The listing builds one solid part. Answer for the finished solid, in the listing's coordinates (mm). A direction names the side the tool comes from. Round coordinates to 2 decimals unless told otherwise and drop trailing zeros. Write each loop counter-clockwise with the first axis right and the second up, starting at its lowest first coordinate (ties: lowest second). Pieces come first, ordered by that corner, then holes.
from build123d import *

# Parameters (mm, degrees)
EXTRUDE_START             = -26
SKETCH_1_W                = 14
SKETCH_1_H                = 1.5
EXTRUDE_241_DEPTH         = 52
SKETCH_2_W                = 5
SKETCH_2_H                = 3
EXTRUDE_321_DEPTH         = 8
SKETCH_3_R                = 3
EXTRUDE_392_DEPTH         = 8
EXTRUDE_START_2           = 18
SKETCH_4_W                = 5
SKETCH_4_H                = 3
EXTRUDE_4_DEPTH           = 8
SKETCH_5_R                = 3
EXTRUDE_5_DEPTH           = 8
D3P2_START                = -28
SKETCH_6_R                = 1.6
D3P2_DEPTH                = 56
CUT_EXTRUDE_M3_DEPTH      = 100
CUT_EXTRUDE_M3_DEPTH_BACK = 100
SKETCH_7_R                = 1.6
CUT_EXTRUDE_3_DEPTH       = 100
CUT_EXTRUDE_3_DEPTH_BACK  = 100
SKETCH_8_R                = 1.6


with BuildPart() as part:
    # 草图1 → Extrude 241 (new body)
    with BuildSketch(Plane.XY.offset(EXTRUDE_START)):
        with Locations((-11, -2.25)):
            Rectangle(SKETCH_1_W, SKETCH_1_H)
    extrude(amount=EXTRUDE_241_DEPTH)

    # 草图2 → Extrude 321 (add)
    with BuildSketch(Plane.XY.offset(EXTRUDE_START)):
        with Locations((-2.5, -1.5)):
            Rectangle(SKETCH_2_W, SKETCH_2_H)
    extrude(amount=EXTRUDE_321_DEPTH)

    # 草图3 → Extrude 392 (add)
    with BuildSketch(Plane.XY.offset(EXTRUDE_START)):
        Circle(SKETCH_3_R)
    extrude(amount=EXTRUDE_392_DEPTH)

    # 草图4 → 凸台-拉伸4 (add)
    with BuildSketch(Plane.XY.offset(EXTRUDE_START_2)):
        with Locations((-2.5, -1.5)):
            Rectangle(SKETCH_4_W, SKETCH_4_H)
    extrude(amount=EXTRUDE_4_DEPTH)

    # 草图5 → 凸台-拉伸5 (add)
    with BuildSketch(Plane.XY.offset(EXTRUDE_START_2)):
        Circle(SKETCH_5_R)
    extrude(amount=EXTRUDE_5_DEPTH)

    # 草图6 → D3p2转轴通孔 (cut)
    with BuildSketch(Plane.XY.offset(D3P2_START)):
        Circle(SKETCH_6_R)
    extrude(amount=D3P2_DEPTH, mode=Mode.SUBTRACT)

    # 草图7 → 底板M3安装孔 (cut, two sides: drawn at the far end of the back side and taken through both)
    with BuildSketch(Plane(origin=(0, 0, 0), x_dir=(1, 0, 0), z_dir=(0, 1, 0)).offset(-CUT_EXTRUDE_M3_DEPTH_BACK)):
        with Locations(Location((-12, 22, 0), (0, 0, 270))):
            Circle(SKETCH_7_R)
    extrude(amount=CUT_EXTRUDE_M3_DEPTH + CUT_EXTRUDE_M3_DEPTH_BACK, mode=Mode.SUBTRACT)

    # 草图8 → 切除-拉伸3 (cut, two sides: drawn at the far end of the back side and taken through both)
    with BuildSketch(Plane(origin=(0, 0, 0), x_dir=(1, 0, 0), z_dir=(0, 1, 0)).offset(-CUT_EXTRUDE_3_DEPTH_BACK)):
        with Locations(Location((-12, -22, 0), (0, 0, 270))):
            Circle(SKETCH_8_R)
    extrude(amount=CUT_EXTRUDE_3_DEPTH + CUT_EXTRUDE_3_DEPTH_BACK, mode=Mode.SUBTRACT)


solid = part.part
1. For a pull along X with two mould halves and no side action, classify faces 1 (the face through (-13.42, -2.26, 22.74)), 2 (the face through (-1.27, -0.97, -22.06)), 3 (the face through (-5, -1, 22)), 4 (the face through (-5, -2, 26)) as released by +X, released by -X, zero draft, split by the parting line, or undercut.
Geometry says:
face 1: undercut
face 2: undercut
face 3: released by -X
face 4: zero draft
2. Section D-D on z = 11 is taken. Determine the outline of the cut face in (x, y), plus the area to 3 significant figures.
Geometry says:
outline: (-18, -3) - (-4, -3) - (-4, -1.5) - (-18, -1.5) - close
area: 21.0 mm2
3. A tool of negligible diameter and unlimited length cuts with its end or side. For faces 5 (the face through (-11, -3, 0)), 6 (the face through (-4, -2, 0)), 7 (the face through (-4, 0, 22)), from which of +Z, -Z, +X, -X, +Y, -Y can it reach the whole face along a straight path? Write none if from no direction.
Geometry says:
face 5: +Z, -Z, +X, -X, -Y
face 6: +X, +Y, -Y
face 7: +Z, -Z, -X, +Y
4. Section A-A on z = 22 is taken. Determine the outline of the cut face in (x, y), plus the area to 3 significant figures.
Geometry says:
outline: (-18, -3) - (-13.6, -3) - (-13.6, -1.5) - (-18, -1.5) - close; (-10.4, -3) - (0, -3) arc R3 ccw (long way) to (-3, 0) - (-5, 0) - (-5, -1.5) - (-10.4, -1.5) - close; hole circle Ø3.2 at (0, 0)
area: 42.9 mm2
5. Section C-C on x = -9.25 is taken. Determine the outline of the cut face in (y, z), plus the area to 3 significant figures.
Geometry says:
outline: (-3, -26) - (-1.5, -26) - (-1.5, 26) - (-3, 26) - close
area: 78.0 mm2
6. Section B-B on x = -12 is taken. Determine the outline of the cut face in (y, z).
Geometry says:
outline: (-3, -26) - (-1.5, -26) - (-1.5, -23.6) - (-3, -23.6) - close; (-3, -20.4) - (-1.5, -20.4) - (-1.5, 20.4) - (-3, 20.4) - close; (-3, 23.6) - (-1.5, 23.6) - (-1.5, 26) - (-3, 26) - close
7. Straight lines are drawn through the part: line 1 along Z through (x, y) = (-12, -2.25); line 2 along Y through (x, z) = (0, -24); line 3 along Y through (x, z) = (-11.75, 13.5). For each, find the intervals that lie inside material, in ascending order.
Geometry says:
line 1: z = -26 to -23.6, -20.4 to 20.4, 23.6 to 26
line 2: y = -3 to -1.6, 1.6 to 3
line 3: y = -3 to -1.5
8. Given pin 1 (0.6 mm diameter, centred on x = -4.5, z = 20.5, fed in from +Y); pin 2 (2 mm diameter, centred on x = -5.5, z = 2, fed in from +Y); pin 3 (0.8 mm diameter, centred on y = -2.5, z = 4.5, fed in from +X), each flat-ended and moving along its own axis, determine where each tip first touches the part or whether it passes through.
Geometry says:
pin 1: stops at y = 0
pin 2: stops at y = -1.5
pin 3: stops at x = -4
